Can you work these out from the model? Positions are in its coordinate system, mm. Face numbers are marked on the shaded views. A direction names the side the tool comes from. Give positions to 0.01 mm unless a question says otherwise; leave off trailing zeros. Write each loop counter-clockwise with the first axis right and the second up, starting at its lowest first coordinate (ties: lowest second). Pieces come first, ordered by that corner, then holes. Notation, with made-up numbers: (63.5, 15) - (77.5, 15) arc R31 ccw to (77.5, 51) - close; hole circle Ø6 at (4, 23.5). An arc over 180 degrees is marked (long way). Return JSON: item names as keys, results as strings. Group by question number.
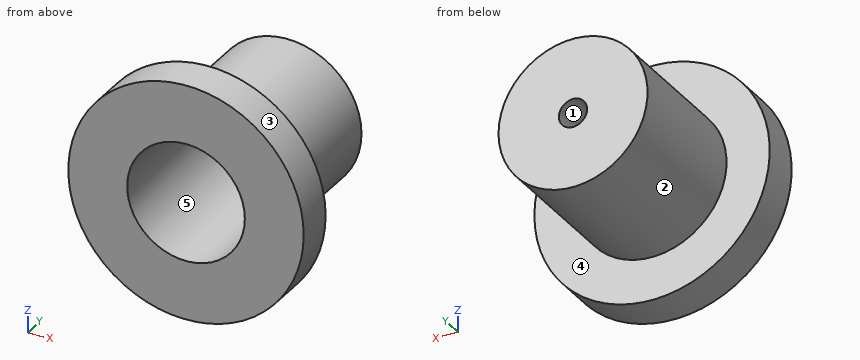
from build123d import *

# Parameters (mm, degrees)
SKETCH2_R            = 15
BOSS_EXTRUDE1_DEPTH  = 5
SKETCH3_R            = 9.5
BOSS_EXTRUDE2_DEPTH  = 18
SKETCH4_R            = 7.5
CUT_EXTRUDE1_DEPTH   = 18
M3_CLEARANCE_HOLE1_D = 3.6


with BuildPart() as part:
    # Sketch2 → Boss-Extrude1 (new body)
    with BuildSketch(Plane(origin=(0, 0, 0), x_dir=(1, 0, 0), z_dir=(0, 1, 0))):
        Circle(SKETCH2_R)
    extrude(amount=BOSS_EXTRUDE1_DEPTH)

    # Sketch3 → Boss-Extrude2 (add)
    with BuildSketch(Plane(origin=(0, 5, 0), x_dir=(1, 0, 0), z_dir=(0, 1, 0))):
        Circle(SKETCH3_R)
    extrude(amount=BOSS_EXTRUDE2_DEPTH)

    # Sketch4 → Cut-Extrude1 (cut)
    with BuildSketch(Plane.XZ):
        Circle(SKETCH4_R)
    extrude(amount=-CUT_EXTRUDE1_DEPTH, mode=Mode.SUBTRACT)

    # M3 Clearance Hole1 (through all)
    with Locations(Plane(origin=(0, 23, 0), x_dir=(1, 0, 0), z_dir=(0, 1, 0))):
        with Locations((0, 0)):
            Hole(M3_CLEARANCE_HOLE1_D / 2)


solid = part.part
1) Will these pins go through, and if not, where does the flat tip stop? pin 1 Ø12 at (y, z) = (12.5, -5) entering from -X; pin 2 Ø2 at (x, z) = (2, 12) entering from +Y; pin 3 Ø3 at (x, y) = (-5, 17) entering from -Z.
2) On a 3-axis mill with a long thin cutter (end or side, diameter ignored), from which of +Z, -Z, +X, -X, +Y, -Y can I reach the whole of each face in a straight line? I mean the marked faces 1 and 2. Say none if no direction works.
3) We'd pull the mould along Z, two halves only. Please class the marked faces 3, 4 and 5: pulls with the +Z half, pulls with the -Z half, needs draft (parallel to the pull), parting line crosses it, or undercut.
4) Imagine slicing it at C-C, the plane y = 3. Write out the boundary of the cut face in (x, z).
5) I need wall thicknesses on line 1 along Z through (x, y) = (0, 19.85); line 2 along X through (y, z) = (13, 0.25). Which ranges of each line are inside material? Lowest first, please.
6) Imagine slicing it at B-B, the plane z = 0. Write out the boundary of the cut face in (x, y).
7) Imagine slicing it at D-D, the plane x = -3. Write out the boundary of the cut face in (y, z).
8) Imagine slicing it at A-A, the plane x = 0. Write out the boundary of the cut face in (y, z).
Resolved:
{
 "1": {"pin 1": "x = -9.5", "pin 2": "y = 5", "pin 3": "z = -8.83"},
 "2": {"face 1": "+Y, -Y", "face 2": "+Y"},
 "3": {"face 3": "parting line crosses it", "face 4": "needs draft", "face 5": "undercut"},
 "4": {"outline": "circle Ø30 at (0, 0); hole circle Ø15 at (0, 0)"},
 "5": {"line 1": "-9.5 to -1.8, 1.8 to 9.5", "line 2": "-9.5 to -7.5, 7.5 to 9.5"},
 "6": {"outline": "(-15, 0) - (-7.5, 0) - (-7.5, 18) - (-1.8, 18) - (-1.8, 23) - (-9.5, 23) - (-9.5, 5) - (-15, 5) - close; (1.8, 18) - (7.5, 18) - (7.5, 0) - (15, 0) - (15, 5) - (9.5, 5) - (9.5, 23) - (1.8, 23) - close"},
 "7": {"outline": "(0, -14.7) - (5, -14.7) - (5, -9.01) - (23, -9.01) - (23, 9.01) - (5, 9.01) - (5, 14.7) - (0, 14.7) - (0, 6.87) - (18, 6.87) - (18, -6.87) - (0, -6.87) - close"},
 "8": {"outline": "(0, -15) - (5, -15) - (5, -9.5) - (23, -9.5) - (23, -1.8) - (18, -1.8) - (18, -7.5) - (0, -7.5) - close; (0, 7.5) - (18, 7.5) - (18, 1.8) - (23, 1.8) - (23, 9.5) - (5, 9.5) - (5, 15) - (0, 15) - close"}
}
